Build history of the part. All positions in model axes, mm. Round coordinates to 2 decimals unless told otherwise and drop trailing zeros. Loops run counter-clockwise (first coordinate to the right, second up) from the corner with the lowest first, then second, coordinate; pieces in that order, holes last. Notation, with made-up numbers: (-9.5, 8.5) - (37.5, 8.5) arc R13 ccw to (37.5, 17.5) - close; hole circle Ø1 at (77, 33.25). An arc over 180 degrees is marked (long way). Use a Markdown table: item, result.
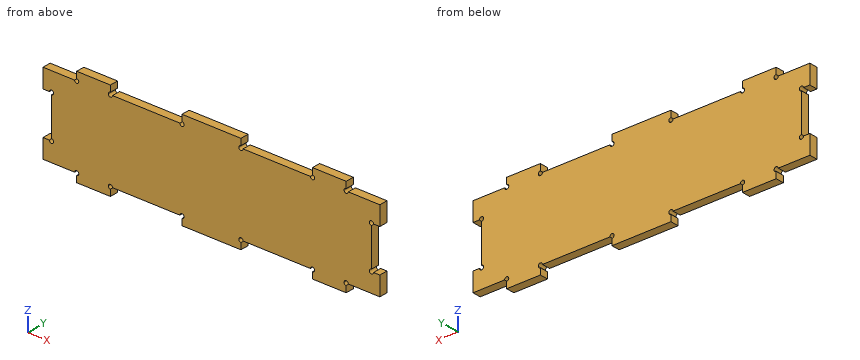
from build123d import *

# Parameters (mm, degrees)
F1_DEPTH = 6.35


with BuildPart() as f1:
    # F0 (on Front) → F1 (new body)
    with BuildSketch(Plane.XZ):
        with BuildLine():
            ThreePointArc((-96.566791, 22.286435), (-95.444259, 21.821467), (-94.979291, 20.698935))
            Line((-94.979291, 20.698935), (-72.754291, 20.698935))
            ThreePointArc((-72.754291, 20.698935), (-72.289323, 21.821467), (-71.166791, 22.286435))
            Line((-71.166791, 22.286435), (-71.166791, 27.048935))
            Line((-71.166791, 27.048935), (-96.566791, 27.048935))
            Line((-96.566791, 27.048935), (-96.566791, 22.286435))
        make_face()
        with BuildLine():
            Line((-72.754291, 20.698935), (-94.979291, 20.698935))
            ThreePointArc((-94.979291, 20.698935), (-96.566791, 19.111435), (-98.154291, 20.698935))
            Line((-98.154291, 20.698935), (-121.966791, 20.698935))
            Line((-121.966791, 20.698935), (-121.966791, 6.411435))
            Line((-121.966791, 6.411435), (-117.204291, 6.411435))
            ThreePointArc((-117.204291, 6.411435), (-115.616791, 7.998935), (-114.029291, 6.411435))
            ThreePointArc((-114.029291, 6.411435), (-114.494259, 5.288903), (-115.616791, 4.823935))
            Line((-115.616791, 4.823935), (-115.616791, -23.751065))
            ThreePointArc((-115.616791, -23.751065), (-114.494259, -24.216033), (-114.029291, -25.338565))
            ThreePointArc((-114.029291, -25.338565), (-115.616791, -26.926065), (-117.204291, -25.338565))
            Line((-117.204291, -25.338565), (-121.966791, -25.338565))
            Line((-121.966791, -25.338565), (-121.966791, -39.626065))
            Line((-121.966791, -39.626065), (-98.154291, -39.626065))
            ThreePointArc((-98.154291, -39.626065), (-96.566791, -38.038565), (-94.979291, -39.626065))
            Line((-94.979291, -39.626065), (-72.754291, -39.626065))
            ThreePointArc((-72.754291, -39.626065), (-71.166791, -38.038565), (-69.579291, -39.626065))
            Line((-69.579291, -39.626065), (-18.779291, -39.626065))
            ThreePointArc((-18.779291, -39.626065), (-17.191791, -38.038565), (-15.604291, -39.626065))
            Line((-15.604291, -39.626065), (25.670709, -39.626065))
            ThreePointArc((25.670709, -39.626065), (27.258209, -38.038565), (28.845709, -39.626065))
            Line((28.845709, -39.626065), (79.645709, -39.626065))
            ThreePointArc((79.645709, -39.626065), (81.233209, -38.038565), (82.820709, -39.626065))
            Line((82.820709, -39.626065), (105.045709, -39.626065))
            ThreePointArc((105.045709, -39.626065), (106.633209, -38.038565), (108.220709, -39.626065))
            Line((108.220709, -39.626065), (132.033209, -39.626065))
            Line((132.033209, -39.626065), (132.033209, -25.338565))
            Line((132.033209, -25.338565), (127.270709, -25.338565))
            ThreePointArc((127.270709, -25.338565), (124.560677, -26.461097), (125.683209, -23.751065))
            Line((125.683209, -23.751065), (125.683209, 4.823935))
            ThreePointArc((125.683209, 4.823935), (124.560677, 7.533967), (127.270709, 6.411435))
            Line((127.270709, 6.411435), (132.033209, 6.411435))
            Line((132.033209, 6.411435), (132.033209, 20.698935))
            Line((132.033209, 20.698935), (108.220709, 20.698935))
            ThreePointArc((108.220709, 20.698935), (106.633209, 19.111435), (105.045709, 20.698935))
            Line((105.045709, 20.698935), (82.820709, 20.698935))
            ThreePointArc((82.820709, 20.698935), (81.233209, 19.111435), (79.645709, 20.698935))
            Line((79.645709, 20.698935), (28.845709, 20.698935))
            ThreePointArc((28.845709, 20.698935), (27.258209, 19.111435), (25.670709, 20.698935))
            Line((25.670709, 20.698935), (-15.604291, 20.698935))
            ThreePointArc((-15.604291, 20.698935), (-17.191791, 19.111435), (-18.779291, 20.698935))
            Line((-18.779291, 20.698935), (-69.579291, 20.698935))
            ThreePointArc((-69.579291, 20.698935), (-71.166791, 19.111435), (-72.754291, 20.698935))
        make_face()
        with BuildLine():
            Line((-17.191791, 27.048935), (-17.191791, 22.286435))
            ThreePointArc((-17.191791, 22.286435), (-16.069259, 21.821467), (-15.604291, 20.698935))
            Line((-15.604291, 20.698935), (25.670709, 20.698935))
            ThreePointArc((25.670709, 20.698935), (26.135677, 21.821467), (27.258209, 22.286435))
            Line((27.258209, 22.286435), (27.258209, 27.048935))
            Line((27.258209, 27.048935), (-17.191791, 27.048935))
        make_face()
        with BuildLine():
            Line((81.233209, 27.048935), (81.233209, 22.286435))
            ThreePointArc((81.233209, 22.286435), (82.355741, 21.821467), (82.820709, 20.698935))
            Line((82.820709, 20.698935), (105.045709, 20.698935))
            ThreePointArc((105.045709, 20.698935), (105.510677, 21.821467), (106.633209, 22.286435))
            Line((106.633209, 22.286435), (106.633209, 27.048935))
            Line((106.633209, 27.048935), (81.233209, 27.048935))
        make_face()
        with BuildLine():
            Line((105.045709, -39.626065), (82.820709, -39.626065))
            ThreePointArc((82.820709, -39.626065), (82.355741, -40.748597), (81.233209, -41.213565))
            Line((81.233209, -41.213565), (81.233209, -45.976065))
            Line((81.233209, -45.976065), (106.633209, -45.976065))
            Line((106.633209, -45.976065), (106.633209, -41.213565))
            ThreePointArc((106.633209, -41.213565), (105.510677, -40.748597), (105.045709, -39.626065))
        make_face()
        with BuildLine():
            Line((25.670709, -39.626065), (-15.604291, -39.626065))
            ThreePointArc((-15.604291, -39.626065), (-16.069259, -40.748597), (-17.191791, -41.213565))
            Line((-17.191791, -41.213565), (-17.191791, -45.976065))
            Line((-17.191791, -45.976065), (27.258209, -45.976065))
            Line((27.258209, -45.976065), (27.258209, -41.213565))
            ThreePointArc((27.258209, -41.213565), (26.135677, -40.748597), (25.670709, -39.626065))
        make_face()
        with BuildLine():
            Line((-72.754291, -39.626065), (-94.979291, -39.626065))
            ThreePointArc((-94.979291, -39.626065), (-95.444259, -40.748597), (-96.566791, -41.213565))
            Line((-96.566791, -41.213565), (-96.566791, -45.976065))
            Line((-96.566791, -45.976065), (-71.166791, -45.976065))
            Line((-71.166791, -45.976065), (-71.166791, -41.213565))
            ThreePointArc((-71.166791, -41.213565), (-72.289323, -40.748597), (-72.754291, -39.626065))
        make_face()
    extrude(amount=F1_DEPTH)


solid = f1.part
Q1. Probe line 1 (X direction, y = -5, z = 24); line 2 (Z direction, x = -96.5, y = -0.25); line 3 (Z direction, x = 73.5, y = -1). List the from-to ranges inside material, lowest first.
Results found:
| item | result |
|---|---|
| line 1 | x = -96.57 to -71.17, -17.19 to 27.26, 81.23 to 106.63 |
| line 2 | z = -45.98 to -41.21, -38.04 to 19.11, 22.29 to 27.05 |
| line 3 | z = -39.63 to 20.7 |
Q2. Cut at A-A, the plane z = -8. List the corners of the cut face in (x, y), plus the area to 3 significant figures.
Results found:
| item | result |
|---|---|
| outline | (-115.62, -6.35) - (125.68, -6.35) - (125.68, 0) - (-115.62, 0) - close |
| area | 1,530 mm2 |
Q3. Drop flat-ended pins along their axis: pin 1 (2.5 mm diameter, centred on y = -4.5, z = 25.5, fed in from +X); pin 2 (1.4 mm diameter, centred on x = -120.5, y = -4, fed in from -Z); pin 3 (1 mm diameter, centred on x = -59, y = -1, fed in from +Z). Give the stop position or say it passes through.
Results found:
| item | result |
|---|---|
| pin 1 | stops at x = 106.63 |
| pin 2 | stops at z = -39.63 |
| pin 3 | stops at z = 20.7 |
Q4. Cut at B-B, the plane x = 42.5. List the corners of the cut face in (y, z).
Results found:
| item | result |
|---|---|
| outline | (-6.35, -39.63) - (0, -39.63) - (0, 20.7) - (-6.35, 20.7) - close |
